from build123d import *

# Parameters (mm, degrees)
SKETCH_1_W          = 45
SKETCH_1_H          = 8
SKETCH_1_R          = 1
EXTRUDE_1_DEPTH     = 1.2
SKETCH_2_W          = 45
SKETCH_2_H          = 30.15
SKETCH_2_R          = 1
SKETCH_2_R_2        = 4.25
EXTRUDE_2_DEPTH     = 1.2
CUT_EXTRUDE_1_DEPTH = 60.007308869
FILLET_2_R          = 8
FILLET_3_R          = 2
EXTRUDE_START       = -1.2
SKETCH_7_R          = 1
SKETCH_7_W          = 45
SKETCH_7_H          = 0.26
EXTRUDE_3_DEPTH     = 1.2
SKETCH_8_W          = 45
SKETCH_8_H          = 0.26
CUT_EXTRUDE_2_DEPTH = 59.24231093
SKETCH_9_R          = 1
CUT_EXTRUDE_3_DEPTH = 59.24231093
SKETCH_10_R         = 4.25
SKETCH_10_R_2       = 1
EXTRUDE_4_DEPTH     = 1.2
SKETCH_11_R         = 4.25
SKETCH_11_R_2       = 1
CUT_EXTRUDE_4_DEPTH = 59.24231093


with BuildPart() as part:
    # ｽｹｯﾁ1 → ﾎﾞｽ - 押し出し1 (new body)
    with BuildSketch(Plane(origin=(0, 0, 0), x_dir=(1, 0, 0), z_dir=(0, 1, 0))):
        with Locations((22.5, 4)):
            Rectangle(SKETCH_1_W, SKETCH_1_H)
        with Locations(Location((2, 3.78, 0), (0, 0, 270))):
            Circle(SKETCH_1_R, mode=Mode.SUBTRACT)
        with Locations(Location((43, 3.78, 0), (0, 0, 90))):
            Circle(SKETCH_1_R, mode=Mode.SUBTRACT)
    extrude(amount=EXTRUDE_1_DEPTH)

    # ｽｹｯﾁ2 → ﾎﾞｽ - 押し出し2 (add)
    with BuildSketch(Plane(origin=(0, 1.2, 0), x_dir=(1, 0, 0), z_dir=(0, 1, 0))):
        with Locations((22.5, 23.075)):
            Rectangle(SKETCH_2_W, SKETCH_2_H)
        with Locations(Location((22.5, 35.15, 0), (0, 0, 270))):
            Circle(SKETCH_2_R, mode=Mode.SUBTRACT)
        with Locations(Location((22.5, 17.1, 0), (0, 0, 270))):
            Circle(SKETCH_2_R_2, mode=Mode.SUBTRACT)
    extrude(amount=-EXTRUDE_2_DEPTH)

    # ｽｹｯﾁ6 → ｶｯﾄ - 押し出し1 (cut, through all)
    with BuildSketch(Plane(origin=(0, 1.2, 0), x_dir=(1, 0, 0), z_dir=(0, 1, 0))):
        Polygon((0, 38.15), (0, 10.130291319), (22.5, 38.15), align=None)
        Polygon((45, 38.15), (22.5, 38.15), (45, 10.130291319), align=None)
    extrude(amount=-CUT_EXTRUDE_1_DEPTH, mode=Mode.SUBTRACT)

    # ﾌｨﾚｯﾄ2
    fillet_2_edges = [part.edges().sort_by_distance(p)[0] for p in [
        (45, 0.6, -10.130291319),
        (0, 0.6, -10.130291319),
    ]]
    fillet(fillet_2_edges, radius=FILLET_2_R)

    # ﾌｨﾚｯﾄ3
    fillet_3_edges = [part.edges().sort_by_distance(p)[0] for p in [
        (22.5, 0.6, -38.15),
    ]]
    fillet(fillet_3_edges, radius=FILLET_3_R)

    # ｽｹｯﾁ7 → ﾎﾞｽ - 押し出し3 (add)
    with BuildSketch(Plane(origin=(0, 1.2, 0), x_dir=(1, 0, 0), z_dir=(0, 1, 0)).offset(EXTRUDE_START)):
        with Locations((2, 3.78)):
            Circle(SKETCH_7_R)
        with Locations((43, 3.78)):
            Circle(SKETCH_7_R)
        with Locations((22.5, 0.13)):
            Rectangle(SKETCH_7_W, SKETCH_7_H)
    extrude(amount=EXTRUDE_3_DEPTH)

    # ｽｹｯﾁ8 → ｶｯﾄ - 押し出し2 (cut, through all)
    with BuildSketch(Plane(origin=(0, 1.2, 0), x_dir=(1, 0, 0), z_dir=(0, 1, 0))):
        with Locations((22.5, 0.13)):
            Rectangle(SKETCH_8_W, SKETCH_8_H)
    extrude(amount=-CUT_EXTRUDE_2_DEPTH, mode=Mode.SUBTRACT)

    # ｽｹｯﾁ9 → ｶｯﾄ - 押し出し3 (cut, through all)
    with BuildSketch(Plane(origin=(0, 1.2, 0), x_dir=(1, 0, 0), z_dir=(0, 1, 0))):
        with Locations(Location((2.3, 4.26, 0), (0, 0, 270))):
            Circle(SKETCH_9_R)
        with Locations(Location((42.7, 4.26, 0), (0, 0, 90))):
            Circle(SKETCH_9_R)
    extrude(amount=-CUT_EXTRUDE_3_DEPTH, mode=Mode.SUBTRACT)

    # ｽｹｯﾁ10 → ﾎﾞｽ - 押し出し4 (add)
    with BuildSketch(Plane(origin=(0, 1.2, 0), x_dir=(1, 0, 0), z_dir=(0, 1, 0))):
        with Locations((22.5, 17.1)):
            Circle(SKETCH_10_R)
        with Locations((22.5, 35.15)):
            Circle(SKETCH_10_R_2)
    extrude(amount=-EXTRUDE_4_DEPTH)

    # ｽｹｯﾁ11 → ｶｯﾄ - 押し出し4 (cut, through all)
    with BuildSketch(Plane(origin=(0, 1.2, 0), x_dir=(1, 0, 0), z_dir=(0, 1, 0))):
        with Locations(Location((22.5, 17.05, 0), (0, 0, 270))):
            Circle(SKETCH_11_R)
        with Locations(Location((22.5, 35.14, 0), (0, 0, 270))):
            Circle(SKETCH_11_R_2)
    extrude(amount=-CUT_EXTRUDE_4_DEPTH, mode=Mode.SUBTRACT)


solid = part.part
Can you work these out from the model? Positions are in its coordinate system, mm. Give positions to 0.01 mm unless a question says otherwise; leave off trailing zeros. Loops run counter-clockwise (first coordinate to the right, second up) from the corner with the lowest first, then second, coordinate; pieces in that order, holes last. Notation, with made-up numbers: M 58,67.5 L 108,67.5 A5 cw 108,74.5 Z; hole C 62.5,82.25 d10. An arc over 180 degrees is marked long. One line per item, written item: value. Start each with the question number.
1) Thinking about a two-plate mould opening in Z: for faces 1 (the face through (21.6, 0.6, -34.7)), 2 (the face through (1.69, 0.61, -5.05)), 3 (the face through (45, 1, -4)), 4 (the face through (33.514, 0.608, -24.434)), which applies, +Z half, -Z half, draft (parallel to the pull), parting line (faces both ways), or undercut?
2) If I drill on line 1 (X direction, y = 0.65, z = -4.26); line 2 (X direction, y = 0.85, z = -35.14); line 3 (X direction, y = 0.8, z = -17.05), over which ranges is the centre line in solid material (lowest first)? Write a range as [from, to].
3) If we section it at C-C, the plane x = 42.7: Write out the boundary of the cut face in (y, z), and give its area (3 significant figures).
4) If we section it at B-B, the plane y = 0.85: Write out the boundary of the cut face in (x, z), and give its area (3 significant figures).
5) If we section it at D-D, the plane z = -4.26: Write out the boundary of the cut face in (x, y).
6) If we section it at A-A, the plane z = -17.05: Write out the boundary of the cut face in (x, y), and give its area (3 significant figures).
Completed:
1. face 1: undercut
1. face 2: undercut
1. face 3: draft
1. face 4: -Z half
2. line 1: x = [0, 1.3], [3.3, 41.7], [43.7, 45]
2. line 2: x = [20.08, 21.5], [23.5, 24.92]
2. line 3: x = [5.56, 18.25], [26.75, 39.44]
3. outline: M 0,-12.99 L 1.2,-12.99 L 1.2,-5.26 L 0,-5.26 Z; M 0,-3.26 L 1.2,-3.26 L 1.2,-0.26 L 0,-0.26 Z
3. area: 12.9 mm^2
4. outline: M 0,-7.32 A8 ccw 1.76,-12.32 L 20.94,-36.21 A2 ccw 24.06,-36.21 L 43.24,-12.32 A8 ccw 45,-7.32 L 45,-0.26 L 0,-0.26 Z; hole C 2.3,-4.26 d2; hole C 22.5,-17.05 d8.5; hole C 22.5,-35.14 d2; hole C 42.7,-4.26 d2
4. area: 1,010 mm^2
5. outline: M 0,0 L 1.3,0 L 1.3,1.2 L 0,1.2 Z; M 3.3,0 L 41.7,0 L 41.7,1.2 L 3.3,1.2 Z; M 43.7,0 L 45,0 L 45,1.2 L 43.7,1.2 Z
6. outline: M 5.56,0 L 18.25,0 L 18.25,1.2 L 5.56,1.2 Z; M 26.75,0 L 39.44,0 L 39.44,1.2 L 26.75,1.2 Z
6. area: 30.5 mm^2
